The listing builds one solid part. Answer for the finished solid, in the listing's coordinates (mm). Give positions to 0.01 mm unless a question says otherwise; leave off trailing zeros. Order: outer loops, then holes, each group sorted by start corner. A loop starts at its lowest first (then second) coordinate and runs counter-clockwise, first axis right, second up. Notation, with made-up numbers: (89, 66) - (108, 66) arc R31 cw to (108, 102) - close; hole circle Ø9 at (2, 17). An arc over 180 degrees is marked (long way). Answer in a Markdown table with one row per item.
from build123d import *

# Parameters (mm, degrees)
SKETCH1_W           = 195.58
SKETCH1_H           = 244.475
BOSS_EXTRUDE1_DEPTH = 2.4
BOSS_EXTRUDE2_DEPTH = 4.5
BOSS_EXTRUDE3_DEPTH = 2
SKETCH4_W           = 2
SKETCH4_H           = 10
CUT_EXTRUDE1_DEPTH  = 2.4
SKETCH5_W           = 2
SKETCH5_H           = 12.7
CUT_EXTRUDE2_DEPTH  = 2.4
SKETCH6_R           = 3.25
CUT_EXTRUDE3_DEPTH  = 316.95890876
SKETCH7_W           = 248.705965207
SKETCH7_H           = 26.677752725
CUT_EXTRUDE4_DEPTH  = 234.430124033


with BuildPart() as part:
    # Sketch1 → Boss-Extrude1 (new body)
    with BuildSketch(Plane.XY):
        with Locations((97.79, 122.2375)):
            Rectangle(SKETCH1_W, SKETCH1_H)
    extrude(amount=BOSS_EXTRUDE1_DEPTH)

    # Sketch2 → Boss-Extrude2 (add)
    with BuildSketch(Plane.XY.offset(2.4)):
        Polygon((195.58, 0), (0, 0), (0, -2), (196.923366415, -2), (197.58, -2), (197.58, 246.475), (195.58, 246.475), (0, 246.475), (0, 244.475), (195.58, 244.475), align=None)
    extrude(amount=-BOSS_EXTRUDE2_DEPTH)

    # Sketch3 → Boss-Extrude3 (add)
    with BuildSketch(Plane(origin=(0, 0, -2.1), x_dir=(-1, 0, 0), z_dir=(0, 0, -1))):
        Polygon((0, -2), (-197.58, -2), (-197.58, 246.475), (0, 246.475), (0, 240.50625), (-195.58, 240.50625), (-195.58, 3.96875), (0, 3.96875), align=None)
    extrude(amount=BOSS_EXTRUDE3_DEPTH)

    # Sketch4 → Cut-Extrude1 (cut)
    with BuildSketch(Plane.XY.offset(2.4)):
        with Locations((6, 236.475)):
            Rectangle(SKETCH4_W, SKETCH4_H)
        with Locations((6, 174.475)):
            Rectangle(SKETCH4_W, SKETCH4_H)
        with Locations((87, 174.475)):
            Rectangle(SKETCH4_W, SKETCH4_H)
        with Locations((87, 236.475)):
            Rectangle(SKETCH4_W, SKETCH4_H)
    extrude(amount=-CUT_EXTRUDE1_DEPTH, mode=Mode.SUBTRACT)

    # Sketch5 → Cut-Extrude2 (cut)
    with BuildSketch(Plane.XY.offset(2.4)):
        Polygon((162.7175, 239.475), (190.58, 239.475), (190.58, 241.475), (192.58, 241.475), (192.58, 228.775), (190.58, 228.775), (190.58, 144.225), (139.78, 144.225), (139.78, 239.475), (132.7175, 239.475), (132.7175, 241.475), (162.7175, 241.475), align=None)
        with Locations((103.855, 235.125)):
            Rectangle(SKETCH5_W, SKETCH5_H)
    extrude(amount=-CUT_EXTRUDE2_DEPTH, mode=Mode.SUBTRACT)

    # Sketch6 → Cut-Extrude3 (cut, through all)
    with BuildSketch(Plane.XY.offset(2.4)):
        with Locations((165.18, 120.975)):
            Circle(SKETCH6_R)
        with Locations((165.18, 100.975)):
            Circle(SKETCH6_R)
        with Locations((165.18, 80.975)):
            Circle(SKETCH6_R)
        with Locations((165.18, 60.975)):
            Circle(SKETCH6_R)
        with Locations((165.18, 40.975)):
            Circle(SKETCH6_R)
    extrude(amount=-CUT_EXTRUDE3_DEPTH, mode=Mode.SUBTRACT)

    # Sketch7 → Cut-Extrude4 (cut, through all)
    with BuildSketch(Plane(origin=(0, 122.2375, 0), x_dir=(1, 0, 0), z_dir=(0, 1, 0))):
        with Locations((112.749873787, 1.388723817)):
            Rectangle(SKETCH7_W, SKETCH7_H)
    extrude(amount=-CUT_EXTRUDE4_DEPTH, mode=Mode.SUBTRACT)


solid = part.part
Item 1: Find section D-D on x = 51. Write down the section's boundary in (y, z) (1 decimal).
Answer block:
| item | result |
|---|---|
| outline | (122.2, 0) - (244.5, 0) - (244.5, -2.1) - (240.5, -2.1) - (240.5, -4.1) - (246.5, -4.1) - (246.5, 2.4) - (122.2, 2.4) - close |
Item 2: Determine the mould class of faces 1 (the face through (96, 243, -2.1)), 2 (the face through (98, 244, -4.1)), 3 (the face through (0, 185, 1)) for opening direction Z: pulls with the +Z half, pulls with the -Z half, needs draft (parallel to the pull), parting line crosses it, or undercut.
Answer block:
| item | result |
|---|---|
| face 1 | undercut |
| face 2 | pulls with the -Z half |
| face 3 | needs draft |
Item 3: Each of these flat-tipped pins is pushed along its axis until it touches: P1, Ø3, axis at x = 46.5, z = -0.5, coming from the -Y side; P2, Ø6, axis at x = 61.5, y = 187.5, coming from the -Z side; P3, Ø1.5, axis at x = 105, z = -2, coming from the -Y side. Where does it stop, or does it pass through?
Answer block:
| item | result |
|---|---|
| P1 | y = 122.24 |
| P2 | z = 0 |
| P3 | y = 240.51 |
Item 4: Find section A-A on y = 207. Write down the section's boundary in (x, z).
Answer block:
| item | result |
|---|---|
| outline | (0, 0) - (139.78, 0) - (139.78, 2.4) - (0, 2.4) - close; (190.58, 0) - (195.58, 0) - (195.58, -4.1) - (197.58, -4.1) - (197.58, 2.4) - (190.58, 2.4) - close |
Item 5: Consider line 1 (X direction, y = 202, z = 1.5); line 2 (Z direction, x = 102.5, y = 227); line 3 (Y direction, x = 162, z = -0.75) (3 decimals). Determine where each line is inside the solid, lowest interval first.
Answer block:
| item | result |
|---|---|
| line 1 | 0 to 139.78, 190.58 to 197.58 |
| line 2 | 0 to 2.4 |
| line 3 | 244.475 to 246.475 |
Item 6: Find section C-C on y = 234. Write down the section's boundary in (x, z) (3 decimals), then the cut area to 3 significant figures.
Answer block:
| item | result |
|---|---|
| outline | (0, 0) - (5, 0) - (5, 2.4) - (0, 2.4) - close; (7, 0) - (86, 0) - (86, 2.4) - (7, 2.4) - close; (88, 0) - (102.855, 0) - (102.855, 2.4) - (88, 2.4) - close; (104.855, 0) - (139.78, 0) - (139.78, 2.4) - (104.855, 2.4) - close; (192.58, 0) - (195.58, 0) - (195.58, -4.1) - (197.58, -4.1) - (197.58, 2.4) - (192.58, 2.4) - close |
| area | 341 mm² |
Item 7: Find section B-B on x = 179. Write down the section's boundary in (y, z) (1 decimal).
Answer block:
| item | result |
|---|---|
| outline | (122.2, 0) - (144.2, 0) - (144.2, 2.4) - (122.2, 2.4) - close; (239.5, 0) - (244.5, 0) - (244.5, -2.1) - (240.5, -2.1) - (240.5, -4.1) - (246.5, -4.1) - (246.5, 2.4) - (239.5, 2.4) - close |
